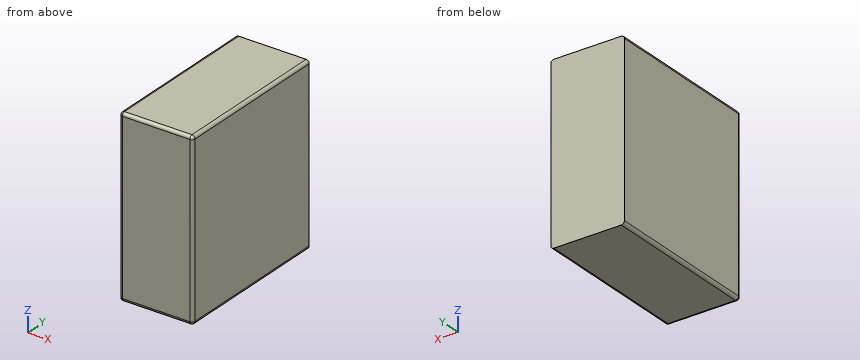
Autodesk Inventor part; units mm, degrees
ref_plane "YZ Plane" through (0, 0, 0) normal (1, 0, 0) x (0, 1, 0)
ref_plane "XZ Plane" through (0, 0, 0) normal (0, 1, 0) x (-1, 0, 0)
ref_plane "XY Plane" through (0, 0, 0) normal (0, 0, 1) x (1, 0, 0)
sketch "Sketch1" plane through (0, 0, 0) normal (1, 0, 0) x (0, 1, 0)
  line L0 (0, 0) -> (167.132, 0)
  line L1 (167.132, 0) -> (167.132, -180.34)
  line L2 (167.132, -180.34) -> (0, -180.34)
  line L3 (0, -180.34) -> (0, 0)
  dimension "d0" = 167.132
  dimension "d1" = 180.34
extrude "Extrusion1" add sketch "Sketch1" along normal blind 76.2
fillet "Fillet1" radius 3.175 8 edges at (76.2, 83.566, 0) (0, 83.566, 0) (76.2, 83.566, -180.34) (0, 83.566, -180.34) (38.1, 0, -180.34) (76.2, 0, -90.17) (38.1, 0, 0) (0, 0, -90.17)
shell "Shell1" thickness 10.16 removed faces 0
properties part number "Battery" material "Concrete"
CAD build for the part. Positions are in the model's coordinates, mm. Coordinates: 2 decimals unless noted, no trailing zeros. Loops run counter-clockwise (first coordinate to the right, second up) from the corner with the lowest first, then second, coordinate; pieces in that order, holes last. Notation, with made-up numbers: (57.5, 31.25) - (97.5, 31.25) arc R19 ccw to (97.5, 63.25) - close; hole circle Ø8 at (58.5, -5.75). An arc over 180 degrees is marked (long way). Use CSV: the item, a comma, the result in double quotes. Start each with the question number.
Q1. Cut at B-B, the plane y = 34. List the corners of the cut face in (x, z) (3 decimals).
Q2. Cut at A-A, the plane x = 46.5. List the corners of the cut face in (y, z) (3 decimals), then the cut area to 3 significant figures.
Q3. Drop a flat-ended pin along its axis: P1, Ø3, axis at x = 31.5, y = 147.5, coming from the +Z side. Give the stop position or say it passes through.
Q4. Probe probe 1 along Z at (x, y) = (30.5, 90); probe 2 along X at (y, z) = (99, -97); probe 3 along Y at (x, z) = (50, -151). List the from-to ranges inside material, lowest first. Write a range as from..to.
Q5. Cut at C-C, the plane z = -63.5. List the corners of the cut face in (x, y) (3 decimals).
Here are the results:
1,outline,"(0, -177.165) arc R3.175 ccw to (3.175, -180.34) - (73.025, -180.34) arc R3.175 ccw to (76.2, -177.165) - (76.2, -3.175) arc R3.175 ccw to (73.025, 0) - (3.175, 0) arc R3.175 ccw to (0, -3.175) - close; hole (10.16, -170.18) - (66.04, -170.18) - (66.04, -10.16) - (10.16, -10.16) - close"
2,outline,"(0, -177.165) arc R3.175 ccw to (3.175, -180.34) - (167.132, -180.34) - (167.132, 0) - (3.175, 0) arc R3.175 ccw to (0, -3.175) - close; hole (10.16, -170.18) - (156.972, -170.18) - (156.972, -10.16) - (10.16, -10.16) - close"
2,area,"6,640 mm2"
3,P1,"z = 0"
4,probe 1,"-180.34..-170.18, -10.16..0"
4,probe 2,"0..10.16, 66.04..76.2"
4,probe 3,"0..10.16, 156.97..167.13"
5,outline,"(0, 3.175) arc R3.175 ccw to (3.175, 0) - (73.025, 0) arc R3.175 ccw to (76.2, 3.175) - (76.2, 167.132) - (0, 167.132) - close; hole (10.16, 10.16) - (66.04, 10.16) - (66.04, 156.972) - (10.16, 156.972) - close"
